The drawing under review shows one solid part. Ordinate dimensions are in mm from its lowest x, y, z. A direction names the side the tool comes from. Coordinates: 2 decimals unless noted, no trailing zeros. Write each loop counter-clockwise with the first axis right and the second up, starting at its lowest first coordinate (ties: lowest second). Pieces come first, ordered by that corner, then holes.
Q1. For probe 1 along Y at (x, z) = (12.7, 2.05) (3 decimals); probe 2 along X at (y, z) = (12.5, 2.5); probe 3 along Y at (x, z) = (14, 6.5), list the stretches that pass through material, from the lowest coordinate up.
Q2. Take a section at C-C (x = 22.5). Give the boundary of the cut face in (y, z) (3 decimals), and give its area (3 significant figures).
Q3. Take a section at D-D (z = 1.5). Give the boundary of the cut face in (x, y) (3 decimals).
Q4. Machinability: for the marked faces 4 and 5, which of the approach directions +Z, -Z, +X, -X, +Y, -Y give a long, thin tool a straight path to every point of the face, cutting with its end or side? Answer none if there is none.
Q5. Take a section at A-A (x = 12.7). Give the boundary of the cut face in (y, z) (3 decimals).
Q6. Take a section at B-B (y = 12.7). Give the boundary of the cut face in (x, z) (3 decimals).
Q7. Insertion check: pin 1 (7 mm diameter, centred on x = 12.7, y = 22.225, fed in from +Z); pin 2 (4 mm diameter, centred on y = 20, z = 6, fed in from +X); pin 3 (4 mm diameter, centred on x = 22, y = 9.5, fed in from +Z) (3 decimals); pin 4 (6 mm diameter, centred on y = 17, z = 8.5, fed in from +X). Each pin has a flat end and moves straight along its axis. Give the tip position at first contact, or say it passes through.
Q8. Mouldability with a two-part tool opening along Y and no side actions: class the marked faces 1, 2 and 3 as pulls with the +Y half, pulls with the -Y half, needs draft (parallel to the pull), parting line crosses it, or undercut.
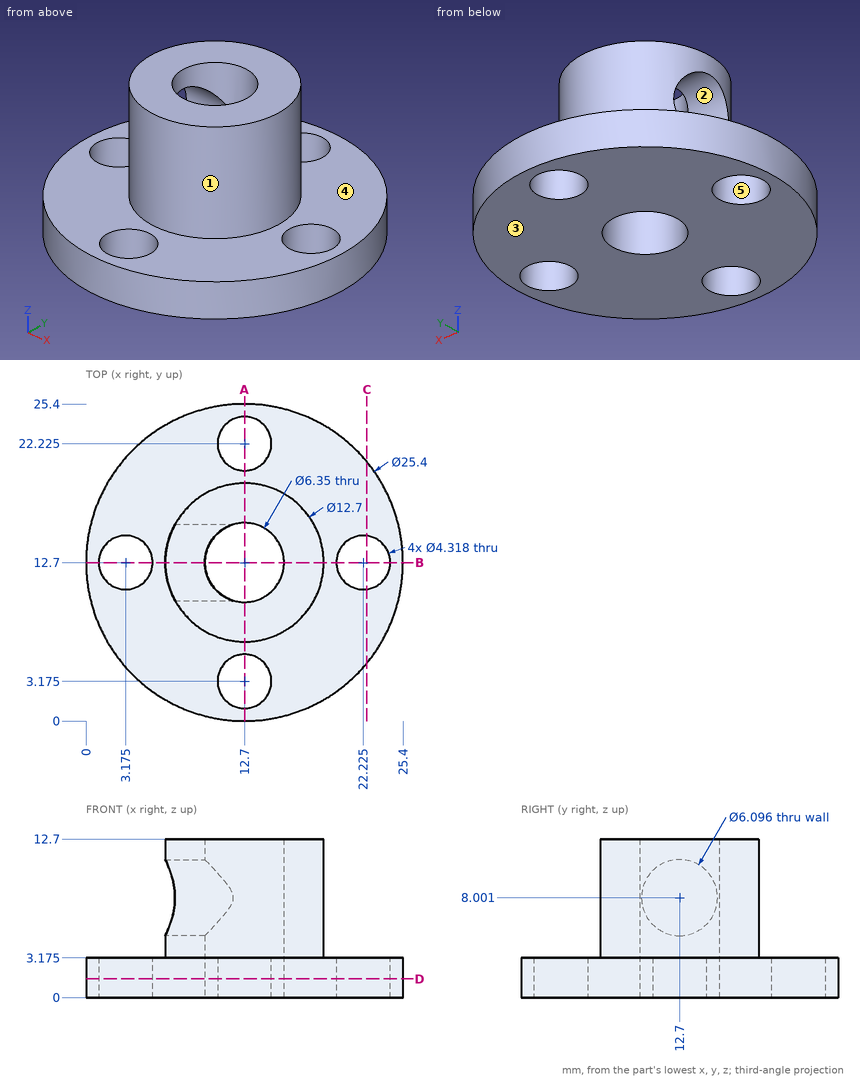
Response:
1. probe 1: y = 0 to 1.016, 5.334 to 9.525, 15.875 to 20.066, 24.384 to 25.4
1. probe 2: x = 0 to 1.03, 5.32 to 9.53, 15.87 to 20.08, 24.37 to 25.4
1. probe 3: y = 6.48 to 9.8, 15.6 to 18.92
2. outline: (4.622, 0) - (10.559, 0) - (10.559, 3.175) - (4.622, 3.175) - close; (14.841, 0) - (20.778, 0) - (20.778, 3.175) - (14.841, 3.175) - close
2. area: 37.7 mm2
3. outline: circle Ø25.4 at (12.7, 12.7); hole circle Ø4.318 at (3.175, 12.7); hole circle Ø6.35 at (12.7, 12.7); hole circle Ø4.318 at (12.7, 3.175); hole circle Ø4.318 at (12.7, 22.225); hole circle Ø4.318 at (22.225, 12.7)
4. face 4: +Z
4. face 5: +Z, -Z
5. outline: (0, 0) - (1.016, 0) - (1.016, 3.175) - (0, 3.175) - close; (5.334, 0) - (9.525, 0) - (9.525, 12.7) - (6.35, 12.7) - (6.35, 3.175) - (5.334, 3.175) - close; (15.875, 0) - (20.066, 0) - (20.066, 3.175) - (19.05, 3.175) - (19.05, 12.7) - (15.875, 12.7) - close; (24.384, 0) - (25.4, 0) - (25.4, 3.175) - (24.384, 3.175) - close
6. outline: (0, 0) - (1.016, 0) - (1.016, 3.175) - (0, 3.175) - close; (5.334, 0) - (9.525, 0) - (9.525, 4.953) - (6.35, 4.953) - (6.35, 3.175) - (5.334, 3.175) - close; (6.35, 11.049) - (9.525, 11.049) - (9.525, 12.7) - (6.35, 12.7) - close; (15.875, 0) - (20.066, 0) - (20.066, 3.175) - (19.05, 3.175) - (19.05, 12.7) - (15.875, 12.7) - close; (24.384, 0) - (25.4, 0) - (25.4, 3.175) - (24.384, 3.175) - close
7. pin 1: stops at z = 12.7
7. pin 2: stops at x = 16.2
7. pin 3: stops at z = 3.175
7. pin 4: stops at x = 18.92
8. face 1: parting line crosses it
8. face 2: undercut
8. face 3: needs draft
